The model under review builds one solid part; all positions refer to its coordinate system, in mm. A direction names the side the tool comes from. Coordinates: 2 decimals unless noted, no trailing zeros. Write each loop counter-clockwise with the first axis right and the second up, starting at its lowest first coordinate (ties: lowest second). Pieces come first, ordered by that corner, then holes. Notation, with made-up numbers: (-39, 9.5) - (-27, 9.5) arc R15 ccw to (-27, 15.5) - close; hole circle Ø1 at (68.25, 27). An arc over 180 degrees is marked (long way). Answer as CSV lines item,"result". Start each with the question number.
```python
from build123d import *

# Parameters (mm, degrees)
SKETCH1_W                                      = 130.554298298
SKETCH1_H                                      = 93.497401401
BOSS_EXTRUDE1_DEPTH                            = 33.046022073
CSK_SLOT_FOR_3_8_FLAT_HEAD_MACHINE_SCREW_DEPTH = 33.046022073


with BuildPart() as part:
    # Sketch1 → Boss-Extrude1 (new body)
    with BuildSketch(Plane(origin=(0, 0, 0), x_dir=(1, 0, 0), z_dir=(0, 1, 0))):
        with Locations((65.277149149, 46.748700701)):
            Rectangle(SKETCH1_W, SKETCH1_H)
    extrude(amount=BOSS_EXTRUDE1_DEPTH)

    # CSK SLOT for 3/8 Flat Head Machine Screw1: read off the stored shape, not the designer's step
    # CSK SLOT for 3_8 Flat Head Machine S 2 → CSK SLOT for 3/8 Flat Head Machine Screw1 (cut)
    with BuildSketch(Plane(origin=(0, 0, 0), x_dir=(1, 0, 0), z_dir=(0, 1, 0))):
        with BuildLine():
            Line((30.486575013, 20.328472109), (30.486575013, 33.028472109))
            ThreePointArc((30.486575013, 33.028472109), (25.444675013, 38.070372109), (20.402775013, 33.028472109))
            Line((20.402775013, 33.028472109), (20.402775013, 20.328472109))
            ThreePointArc((20.402775013, 20.328472109), (25.444675013, 15.286572109), (30.486575013, 20.328472109))
        make_face()
        with BuildLine():
            Line((69.908405086, 23.408302584), (69.908405086, 36.108302584))
            ThreePointArc((69.908405086, 36.108302584), (64.866505086, 41.150202584), (59.824605086, 36.108302584))
            Line((59.824605086, 36.108302584), (59.824605086, 23.408302584))
            ThreePointArc((59.824605086, 23.408302584), (64.866505086, 18.366402584), (69.908405086, 23.408302584))
        make_face()
        with BuildLine():
            Line((104.197184368, 49.4842006), (104.197184368, 62.1842006))
            ThreePointArc((104.197184368, 62.1842006), (99.155284368, 67.2261006), (94.113384368, 62.1842006))
            Line((94.113384368, 62.1842006), (94.113384368, 49.4842006))
            ThreePointArc((94.113384368, 49.4842006), (99.155284368, 44.4423006), (104.197184368, 49.4842006))
        make_face()
        with BuildLine():
            Line((40.547354563, 56.670471707), (40.547354563, 69.370471707))
            ThreePointArc((40.547354563, 69.370471707), (35.505454563, 74.412371707), (30.463554563, 69.370471707))
            Line((30.463554563, 69.370471707), (30.463554563, 56.670471707))
            ThreePointArc((30.463554563, 56.670471707), (35.505454563, 51.628571707), (40.547354563, 56.670471707))
        make_face()
    extrude(amount=CSK_SLOT_FOR_3_8_FLAT_HEAD_MACHINE_SCREW_DEPTH, mode=Mode.SUBTRACT)

    # CSK SLOT for 3_8 Flat Head Machine S 3: loft between two sections, ruled curve by curve
    csk_slot_for_3_8_flat_head_machine_s_3_from = [
        Edge.make_three_point_arc((30.486575013, 27.713489321, -33.028472109), (29.009836693, 27.713489321, -36.593633789), (25.444675013, 27.713489321, -38.070372109)),
        Edge.make_three_point_arc((25.444675013, 27.713489321, -38.070372109), (21.879513333, 27.713489321, -36.593633789), (20.402775013, 27.713489321, -33.028472109)),
        Edge.make_three_point_arc((20.402775013, 27.713489321, -20.328472109), (21.879513333, 27.713489321, -16.763310429), (25.444675013, 27.713489321, -15.286572109)),
        Edge.make_three_point_arc((25.444675013, 27.713489321, -15.286572109), (29.009836693, 27.713489321, -16.763310429), (30.486575013, 27.713489321, -20.328472109)),
        Edge.make_line((20.402775013, 27.713489321, -33.028472109), (20.402775013, 27.713489321, -20.328472109)),
        Edge.make_line((30.486575013, 27.713489321, -33.028472109), (30.486575013, 27.713489321, -20.328472109)),
    ]
    csk_slot_for_3_8_flat_head_machine_s_3_to = [
        Edge.make_three_point_arc((35.122075013, 33.046022073, -33.028472109), (32.287630178, 33.046022073, -39.871427273), (25.444675013, 33.046022073, -42.705872109)),
        Edge.make_three_point_arc((25.444675013, 33.046022073, -42.705872109), (18.601719849, 33.046022073, -39.871427273), (15.767275013, 33.046022073, -33.028472109)),
        Edge.make_three_point_arc((15.767275013, 33.046022073, -20.328472109), (18.601719849, 33.046022073, -13.485516945), (25.444675013, 33.046022073, -10.651072109)),
        Edge.make_three_point_arc((25.444675013, 33.046022073, -10.651072109), (32.287630178, 33.046022073, -13.485516945), (35.122075013, 33.046022073, -20.328472109)),
        Edge.make_line((15.767275013, 33.046022073, -33.028472109), (15.767275013, 33.046022073, -20.328472109)),
        Edge.make_line((35.122075013, 33.046022073, -33.028472109), (35.122075013, 33.046022073, -20.328472109)),
    ]
    csk_slot_for_3_8_flat_head_machine_s_3 = Solid(Shell([*[Face.make_surface_from_curves(csk_slot_for_3_8_flat_head_machine_s_3_from[k], csk_slot_for_3_8_flat_head_machine_s_3_to[k]) for k in range(6)], Face(Wire(csk_slot_for_3_8_flat_head_machine_s_3_from)), Face(Wire(csk_slot_for_3_8_flat_head_machine_s_3_to))]))
    add(csk_slot_for_3_8_flat_head_machine_s_3, mode=Mode.SUBTRACT)

    # CSK SLOT for 3_8 Flat Head Machine S 4: loft between two sections, ruled curve by curve
    csk_slot_for_3_8_flat_head_machine_s_4_from = [
        Edge.make_three_point_arc((69.908405086, 27.713489321, -36.108302584), (68.431666766, 27.713489321, -39.673464264), (64.866505086, 27.713489321, -41.150202584)),
        Edge.make_three_point_arc((64.866505086, 27.713489321, -41.150202584), (61.301343406, 27.713489321, -39.673464264), (59.824605086, 27.713489321, -36.108302584)),
        Edge.make_three_point_arc((59.824605086, 27.713489321, -23.408302584), (61.301343406, 27.713489321, -19.843140903), (64.866505086, 27.713489321, -18.366402584)),
        Edge.make_three_point_arc((64.866505086, 27.713489321, -18.366402584), (68.431666766, 27.713489321, -19.843140903), (69.908405086, 27.713489321, -23.408302584)),
        Edge.make_line((59.824605086, 27.713489321, -36.108302584), (59.824605086, 27.713489321, -23.408302584)),
        Edge.make_line((69.908405086, 27.713489321, -36.108302584), (69.908405086, 27.713489321, -23.408302584)),
    ]
    csk_slot_for_3_8_flat_head_machine_s_4_to = [
        Edge.make_three_point_arc((74.543905086, 33.046022073, -36.108302584), (71.70946025, 33.046022073, -42.951257748), (64.866505086, 33.046022073, -45.785702584)),
        Edge.make_three_point_arc((64.866505086, 33.046022073, -45.785702584), (58.023549922, 33.046022073, -42.951257748), (55.189105086, 33.046022073, -36.108302584)),
        Edge.make_three_point_arc((55.189105086, 33.046022073, -23.408302584), (58.023549922, 33.046022073, -16.565347419), (64.866505086, 33.046022073, -13.730902584)),
        Edge.make_three_point_arc((64.866505086, 33.046022073, -13.730902584), (71.70946025, 33.046022073, -16.565347419), (74.543905086, 33.046022073, -23.408302584)),
        Edge.make_line((55.189105086, 33.046022073, -36.108302584), (55.189105086, 33.046022073, -23.408302584)),
        Edge.make_line((74.543905086, 33.046022073, -36.108302584), (74.543905086, 33.046022073, -23.408302584)),
    ]
    csk_slot_for_3_8_flat_head_machine_s_4 = Solid(Shell([*[Face.make_surface_from_curves(csk_slot_for_3_8_flat_head_machine_s_4_from[k], csk_slot_for_3_8_flat_head_machine_s_4_to[k]) for k in range(6)], Face(Wire(csk_slot_for_3_8_flat_head_machine_s_4_from)), Face(Wire(csk_slot_for_3_8_flat_head_machine_s_4_to))]))
    add(csk_slot_for_3_8_flat_head_machine_s_4, mode=Mode.SUBTRACT)

    # CSK SLOT for 3_8 Flat Head Machine S 5: loft between two sections, ruled curve by curve
    csk_slot_for_3_8_flat_head_machine_s_5_from = [
        Edge.make_three_point_arc((104.197184368, 27.713489321, -62.1842006), (102.720446048, 27.713489321, -65.74936228), (99.155284368, 27.713489321, -67.2261006)),
        Edge.make_three_point_arc((99.155284368, 27.713489321, -67.2261006), (95.590122688, 27.713489321, -65.74936228), (94.113384368, 27.713489321, -62.1842006)),
        Edge.make_three_point_arc((94.113384368, 27.713489321, -49.4842006), (95.590122688, 27.713489321, -45.91903892), (99.155284368, 27.713489321, -44.4423006)),
        Edge.make_three_point_arc((99.155284368, 27.713489321, -44.4423006), (102.720446048, 27.713489321, -45.91903892), (104.197184368, 27.713489321, -49.4842006)),
        Edge.make_line((94.113384368, 27.713489321, -62.1842006), (94.113384368, 27.713489321, -49.4842006)),
        Edge.make_line((104.197184368, 27.713489321, -62.1842006), (104.197184368, 27.713489321, -49.4842006)),
    ]
    csk_slot_for_3_8_flat_head_machine_s_5_to = [
        Edge.make_three_point_arc((108.832684368, 33.046022073, -62.1842006), (105.998239532, 33.046022073, -69.027155764), (99.155284368, 33.046022073, -71.8616006)),
        Edge.make_three_point_arc((99.155284368, 33.046022073, -71.8616006), (92.312329203, 33.046022073, -69.027155764), (89.477884368, 33.046022073, -62.1842006)),
        Edge.make_three_point_arc((89.477884368, 33.046022073, -49.4842006), (92.312329203, 33.046022073, -42.641245436), (99.155284368, 33.046022073, -39.8068006)),
        Edge.make_three_point_arc((99.155284368, 33.046022073, -39.8068006), (105.998239532, 33.046022073, -42.641245436), (108.832684368, 33.046022073, -49.4842006)),
        Edge.make_line((89.477884368, 33.046022073, -62.1842006), (89.477884368, 33.046022073, -49.4842006)),
        Edge.make_line((108.832684368, 33.046022073, -62.1842006), (108.832684368, 33.046022073, -49.4842006)),
    ]
    csk_slot_for_3_8_flat_head_machine_s_5 = Solid(Shell([*[Face.make_surface_from_curves(csk_slot_for_3_8_flat_head_machine_s_5_from[k], csk_slot_for_3_8_flat_head_machine_s_5_to[k]) for k in range(6)], Face(Wire(csk_slot_for_3_8_flat_head_machine_s_5_from)), Face(Wire(csk_slot_for_3_8_flat_head_machine_s_5_to))]))
    add(csk_slot_for_3_8_flat_head_machine_s_5, mode=Mode.SUBTRACT)

    # CSK SLOT for 3_8 Flat Head Machine S 6: loft between two sections, ruled curve by curve
    csk_slot_for_3_8_flat_head_machine_s_6_from = [
        Edge.make_three_point_arc((40.547354563, 27.713489321, -69.370471707), (39.070616243, 27.713489321, -72.935633387), (35.505454563, 27.713489321, -74.412371707)),
        Edge.make_three_point_arc((35.505454563, 27.713489321, -74.412371707), (31.940292883, 27.713489321, -72.935633387), (30.463554563, 27.713489321, -69.370471707)),
        Edge.make_three_point_arc((30.463554563, 27.713489321, -56.670471707), (31.940292883, 27.713489321, -53.105310027), (35.505454563, 27.713489321, -51.628571707)),
        Edge.make_three_point_arc((35.505454563, 27.713489321, -51.628571707), (39.070616243, 27.713489321, -53.105310027), (40.547354563, 27.713489321, -56.670471707)),
        Edge.make_line((30.463554563, 27.713489321, -69.370471707), (30.463554563, 27.713489321, -56.670471707)),
        Edge.make_line((40.547354563, 27.713489321, -69.370471707), (40.547354563, 27.713489321, -56.670471707)),
    ]
    csk_slot_for_3_8_flat_head_machine_s_6_to = [
        Edge.make_three_point_arc((45.182854563, 33.046022073, -69.370471707), (42.348409727, 33.046022073, -76.213426871), (35.505454563, 33.046022073, -79.047871707)),
        Edge.make_three_point_arc((35.505454563, 33.046022073, -79.047871707), (28.662499399, 33.046022073, -76.213426871), (25.828054563, 33.046022073, -69.370471707)),
        Edge.make_three_point_arc((25.828054563, 33.046022073, -56.670471707), (28.662499399, 33.046022073, -49.827516543), (35.505454563, 33.046022073, -46.993071707)),
        Edge.make_three_point_arc((35.505454563, 33.046022073, -46.993071707), (42.348409727, 33.046022073, -49.827516543), (45.182854563, 33.046022073, -56.670471707)),
        Edge.make_line((25.828054563, 33.046022073, -69.370471707), (25.828054563, 33.046022073, -56.670471707)),
        Edge.make_line((45.182854563, 33.046022073, -69.370471707), (45.182854563, 33.046022073, -56.670471707)),
    ]
    csk_slot_for_3_8_flat_head_machine_s_6 = Solid(Shell([*[Face.make_surface_from_curves(csk_slot_for_3_8_flat_head_machine_s_6_from[k], csk_slot_for_3_8_flat_head_machine_s_6_to[k]) for k in range(6)], Face(Wire(csk_slot_for_3_8_flat_head_machine_s_6_from)), Face(Wire(csk_slot_for_3_8_flat_head_machine_s_6_to))]))
    add(csk_slot_for_3_8_flat_head_machine_s_6, mode=Mode.SUBTRACT)


solid = part.part
```
(1) The part is to be moulded in two halves that separate along X. For faces 3 (the flat face through (64, 16, -93.497)), 4 (the flat face through (0, 16, -46)), 5 (the cylindrical face through (25.56, 13.66, -38.07)), say which applies: released by +X, released by -X, zero draft, split by the parting line, or undercut.
(2) Wall thickness on line 1 (Z direction, x = 35, y = 26); line 2 (X direction, y = 22.5, z = -30); line 3 (X direction, y = 2.5, z = -51): over which ranges is each line inside the solid? List them lowest first.
(3) Add section B-B on z = -22. Give the number of separate pieces and of enclosed holes in the cut face, then the cut area to 3 significant figures.
(4) Add section A-A on y = 25.5. Give the boundary of the cut face in (x, z), then the cut area to 3 significant figures.
(5) For faces 1 (the flat face through (130.554, 16, -46)), 2 (the flat face through (94.113, 14, -56)), list the 3-axis set-ups (+Z, -Z, +X, -X, +Y, -Y) from which the entire face can be reached by the end or side of a thin tool; tool diameter is ignored.
Reported:
1,face 3,"zero draft"
1,face 4,"released by -X"
1,face 5,"undercut"
2,line 1,"-93.5 to -74.39, -51.65 to 0"
2,line 2,"0 to 20.4, 30.49 to 59.82, 69.91 to 130.55"
2,line 3,"0 to 94.11, 104.2 to 130.55"
3,separate pieces,"3"
3,enclosed holes,"0"
3,area,"3,610 mm²"
4,outline,"(0, -93.5) - (130.55, -93.5) - (130.55, 0) - (0, 0) - close; hole (20.4, -33.03) arc R5.04 ccw to (30.49, -33.03) - (30.49, -20.33) arc R5.04 ccw to (20.4, -20.33) - close; hole (30.46, -69.37) arc R5.04 ccw to (40.55, -69.37) - (40.55, -56.67) arc R5.04 ccw to (30.46, -56.67) - close; hole (59.82, -36.11) arc R5.04 ccw to (69.91, -36.11) - (69.91, -23.41) arc R5.04 ccw to (59.82, -23.41) - close; hole (94.11, -62.18) arc R5.04 ccw to (104.2, -62.18) - (104.2, -49.48) arc R5.04 ccw to (94.11, -49.48) - close"
4,area,"11,400 mm²"
5,face 1,"+Z, -Z, +X, +Y, -Y"
5,face 2,"+Y, -Y"
